Here's how the part is built. I have some questions about the finished solid (model axes, mm). Face numbers are marked on the shaded views. A direction names the side the tool comes from. Coordinates: 2 decimals unless noted, no trailing zeros. Order: outer loops, then holes, each group sorted by start corner. A loop starts at its lowest first (then second) coordinate and runs counter-clockwise, first axis right, second up. Notation, with made-up numbers: (42.25, 39.5) - (52.25, 39.5) arc R8 cw to (52.25, 47.5) - close; hole circle Ø8 at (63.25, -2). An arc over 180 degrees is marked (long way). Answer in a Markdown table with one row per item. Add a question column.
Item 1: On a 3-axis mill with a long thin cutter (end or side, diameter ignored), from which of +Z, -Z, +X, -X, +Y, -Y can I reach the whole of each face in a straight line? I mean the marked faces 1, 2, 3, 4 and 5. Say none if no direction works.
Item 2: If I drill on line 1 along Z through (x, y) = (19.8, 2); line 2 along Y through (x, z) = (18.6, -0.55); line 3 along X through (y, z) = (-2.75, 1.35), over which ranges is the centre line in solid material (lowest first)? Write a range as from..to.
Item 3: I want a section at B-B (x = 18.3). Please give me the cut outline in (y, z), plus the area to 3 significant figures.
Item 4: I want a section at A-A (x = 19.85). Please give me the cut outline in (y, z), plus the area to 3 significant figures.
Item 5: Will this pin go through, and if not, where does the flat tip stop? pin 1 Ø1.5 at (x, y) = (19.5, -3) entering from -Z.
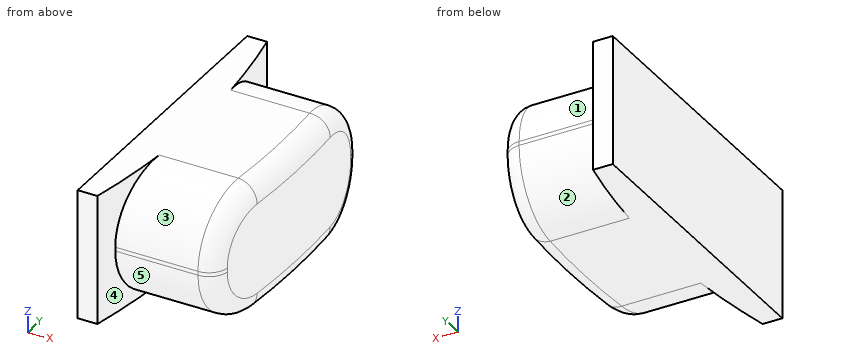
```python
from build123d import *

# Parameters (mm, degrees)
BOSS_EXTRUDE1_DEPTH = 1.65
FILLET1_R           = 1.6
FILLET2_R           = 0.5


with BuildPart() as part:
    # Sketch1 → Boss-Extrude1 (new, symmetric)
    with BuildSketch(Plane.XY):
        with BuildLine():
            Line((18.221141567, 3.2), (20.754758491, 3.2))
            ThreePointArc((20.754758491, 3.2), (21, 0), (20.754758491, -3.2))
            Line((20.754758491, -3.2), (18.221141567, -3.2))
            ThreePointArc((18.221141567, -3.2), (18.165810143, -3.500477375), (18.105524019, -3.8))
            Line((18.105524019, -3.8), (17.605524019, -3.8))
            Line((17.605524019, -3.8), (17.605524019, 3.8))
            Line((17.605524019, 3.8), (18.105524019, 3.8))
            ThreePointArc((18.105524019, 3.8), (18.165810143, 3.500477375), (18.221141567, 3.2))
        make_face()
    extrude(amount=BOSS_EXTRUDE1_DEPTH, both=True)

    # Fillet1
    fillet1_edges = [part.edges().sort_by_distance(p)[0] for p in [
        (19.487950029, 3.2, -1.65),
        (19.487950029, -3.2, 1.65),
        (19.487950029, 3.2, 1.65),
        (19.487950029, -3.2, -1.65),
    ]]
    fillet(fillet1_edges, radius=FILLET1_R)

    # Fillet2
    fillet2_edges = [part.edges().sort_by_distance(p)[0] for p in [
        (21, 0, 1.65),
        (21, 0, -1.65),
        (20.754758491, 3.2, 0),
        (20.754758491, -3.2, 0),
        (20.821763727, 2.730229949, 1.182510681),
        (20.821763726, 2.730229907, -1.182510644),
        (20.821763721, -2.730229944, -1.182510607),
        (20.821763721, -2.730229942, 1.182510608),
    ]]
    fillet(fillet2_edges, radius=FILLET2_R)


solid = part.part
```
Values follow:
| question | item | result |
|---|---|---|
| 1 | face 1 | +Z, +X, +Y |
| 1 | face 2 | -Z, +X, +Y |
| 1 | face 3 | +Z, +X, -Y |
| 1 | face 4 | +X, -Y |
| 1 | face 5 | -Z, +X, -Y |
| 2 | line 1 | z = -1.6..1.6 |
| 2 | line 2 | y = -3.12..3.12 |
| 2 | line 3 | x = 17.61..18.29 |
| 3 | outline | (-3.2, -0.05) arc R1.6 ccw to (-2.71, -1.2) - (-2.71, -1.65) - (2.71, -1.65) - (2.71, -1.2) arc R1.6 ccw to (3.2, -0.05) - (3.2, 0.05) arc R1.6 ccw to (2.71, 1.2) - (2.71, 1.65) - (-2.71, 1.65) - (-2.71, 1.2) arc R1.6 ccw to (-3.2, 0.05) - close |
| 3 | area | 19.5 mm^2 |
| 4 | outline | (-3.2, -0.05) arc R1.6 ccw to (-1.6, -1.65) - (1.6, -1.65) arc R1.6 ccw to (3.2, -0.05) - (3.2, 0.05) arc R1.6 ccw to (1.6, 1.65) - (-1.6, 1.65) arc R1.6 ccw to (-3.2, 0.05) - close |
| 4 | area | 18.9 mm^2 |
| 5 | pin 1 | stops at z = -1.51 |
